```python
from build123d import *

# Parameters (mm, degrees)
SKETCH1_W           = 350
SKETCH1_H           = 40
BOSS_EXTRUDE1_DEPTH = 20
CUT_EXTRUDE1_DEPTH  = 178.270979012
FILLET1_R           = 50
FILLET2_R           = 50
FILLET3_R           = 16.247923
FILLET4_RADIUS      = 20
FILLET4_LENGTH      = 20
SKETCH3_R           = 7.5
SKETCH3_R_2         = 5
CUT_EXTRUDE2_DEPTH  = 178.270979012


with BuildPart() as part:
    # Sketch1 → Boss-Extrude1 (new body)
    with BuildSketch(Plane.XY):
        Rectangle(SKETCH1_W, SKETCH1_H)
    extrude(amount=BOSS_EXTRUDE1_DEPTH)

    # Sketch2 → Cut-Extrude1 (cut, through all)
    with BuildSketch(Plane.XY.offset(20)):
        Polygon((175, 20), (175, 15), (125, 19), (125, 20), align=None)
    cut_extrude1 = extrude(amount=-CUT_EXTRUDE1_DEPTH, mode=Mode.SUBTRACT)

    # Fillet1
    # the kernel refuses this fillet: 50 mm, written as the material it takes off along each edge
    with BuildSketch(Plane(origin=(125, 20, 44.874685928), x_dir=(-1, 0, 0), z_dir=(0, 0, -1))) as fillet1_piece_1:
        with BuildLine():
            CenterArc((9.949874371, -50), FILLET1_R, 90, 11.478340955)
            Line((0, -1), (-0.198997487, -0.02))
            ThreePointArc((-0.198997487, -0.02), (-1, -0.5), (-1, 0))
            Line((-1, 0), (0, 1))
            Line((0, 1), (9.949874371, 1))
            Line((9.949874371, 1), (9.949874371, 0))
        make_face()
    extrude(amount=69.749371855, mode=Mode.SUBTRACT)

    # Mirror3: Cut-Extrude1 across plane
    add(cut_extrude1.mirror(Plane.ZX), mode=Mode.SUBTRACT)

    # Fillet2
    # the kernel refuses this fillet: 50 mm, written as the material it takes off along each edge
    with BuildSketch(Plane(origin=(125, -20, 44.874685928), x_dir=(0, 1, 0), z_dir=(0, 0, -1))) as fillet2_piece_1:
        with BuildLine():
            CenterArc((50, -9.949874371), FILLET2_R, 168.521659045, 11.478340955)
            Line((0, -9.949874371), (-1, -9.949874371))
            Line((-1, -9.949874371), (-1, 0))
            Line((-1, 0), (0, 1))
            ThreePointArc((0, 1), (0.5, 1), (0.02, 0.198997487))
            Line((0.02, 0.198997487), (1, 0))
        make_face()
    extrude(amount=69.749371855, mode=Mode.SUBTRACT)

    # Fillet3
    fillet3_edges = [part.edges().sort_by_distance(p)[0] for p in [
        (175, 15, 10),
        (175, -15, 10),
    ]]
    fillet(fillet3_edges, radius=FILLET3_R)

    # Fillet4: full round fillet: the end face becomes a half cylinder, R = half its width
    fillet4_face = Plane((-175, 0, 10), x_dir=(0, 0, 1), z_dir=(-1, 0, 0))  # on the end face: x along it, z out of the body
    fillet4_slab = fillet4_face.offset(-FILLET4_RADIUS / 2) * Box(FILLET4_LENGTH, 2 * FILLET4_RADIUS, FILLET4_RADIUS, mode=Mode.PRIVATE)  # the body's end, R deep
    fillet4_round = Plane((-155, 0, 10), x_dir=(-1, 0, 0), z_dir=(0, 0, 1)) * Cylinder(FILLET4_RADIUS, FILLET4_LENGTH, mode=Mode.PRIVATE)  # its axis R under the face
    add(fillet4_slab - fillet4_round, mode=Mode.SUBTRACT)

    # Sketch3 → Cut-Extrude2 (cut, through all)
    with BuildSketch(Plane.XY.offset(20)):
        with Locations((-155, 0)):
            Circle(SKETCH3_R)
        with Locations((158.752076555, 0)):
            Circle(SKETCH3_R_2)
    extrude(amount=-CUT_EXTRUDE2_DEPTH, mode=Mode.SUBTRACT)


solid = part.part
```
Verification items for the finished model (mm, model axes). Coordinates: 2 decimals unless noted, no trailing zeros. Write each loop counter-clockwise with the first axis right and the second up, starting at its lowest first coordinate (ties: lowest second). Pieces come first, ordered by that corner, then holes. Notation, with made-up numbers: M -1.5,11 L 35.5,11 A15 ccw 35.5,38 Z; hole C 76,-39.5 d7. An arc over 180 degrees is marked long. Answer as a JSON object with one key per item and string values. Group by question number.
(1) Release check for a two-part mould opening along Y. For faces 1 (the face through (-2, 0, 20)), 2 (the face through (-175, 0, 10)), 3 (the face through (153.757, 0.22, 10.14)), 4 (the face through (-22, -20, 10)) record: +Y half, -Y half, draft (parallel to the pull), parting line (faces both ways), or undercut.
(2) Cross-section at A-A, the plane z = 11.5. State how many separate pieces and enclosed holes the cut face has, and give its area (3 significant figures).
(3) Material ranges on line 1 (X direction, y = 0.5, z = 16); line 2 (Y direction, x = -155, z = 13); line 3 (X direction, y = -3.5, z = 9.25), recorded low to high.
(4) Cross-section at B-B, the plane y = 12.5. Record the cut outline in (x, z), and give its area (3 significant figures).
(5) Gauge pin test, flat ends, axial feed: pin 1 (9 mm diameter, centred on x = 158.75, y = 0, fed in from +Z); pin 2 (2 mm diameter, centred on y = 6.5, z = 8, fed in from +X); pin 3 (10 mm diameter, centred on y = 14.5, z = 4.5, fed in from -X); pin 4 (10 mm diameter, centred on y = 14.5, z = 5.5, fed in from +X). Record the tip position at first contact, or that the pin passes through.
Reply:
{
 "1": {"face 1": "draft", "face 2": "parting line", "face 3": "undercut", "face 4": "-Y half"},
 "2": {"separate pieces": "1", "enclosed holes": "2", "area": "13,200 mm²"},
 "3": {"line 1": "-174.99 to -162.48, -147.52 to 153.78, 163.73 to 174.99", "line 2": "-20 to -7.5, 7.5 to 20", "line 3": "-174.69 to -161.63, -148.37 to 155.18, 162.32 to 174.62"},
 "4": {"outline": "M -170.61,0 L 169.13,0 L 169.13,20 L -170.61,20 Z", "area": "6,790 mm²"},
 "5": {"pin 1": "through", "pin 2": "x = 174.04", "pin 3": "x = -172.6", "pin 4": "x = 171.93"}
}
